Input: part model. Units: mm. Frame: model coordinates. A direction names the side the tool comes from. Coordinates: 2 decimals unless noted, no trailing zeros. Write each loop counter-clockwise with the first axis right and the second up, starting at its lowest first coordinate (ties: lowest second). Pieces come first, ordered by that corner, then holes. Notation, with made-up numbers: (40.25, 19) -> (96.25, 19) arc R14 ccw to (96.25, 38) -> close; hole circle Ø2 at (-15.5, 50). An arc over 180 degrees is marked (long way). One line per question, with ' | ' between items. Start each with the question number.
```python
from build123d import *


with BuildPart() as f1:
    # F0 (on Front) → F1 (revolve)
    with BuildSketch(Plane.XZ):
        with BuildLine():
            Line((0, 1), (0, 0))
            Line((0, 0), (6, 0))
            ThreePointArc((6, 0), (7.5, 2.5), (6, 5))
            ThreePointArc((6, 5), (4.5, 7.5), (6, 10))
            Line((6, 10), (6, 12))
            Line((6, 12), (2.75, 12))
            Line((2.75, 12), (2.75, 1))
            Line((2.75, 1), (0, 1))
        make_face()
    revolve(axis=Axis((0, 0, 0.5), (0, 0, -1)))


solid = f1.part
```
1) Ray query, line 1 (X direction, y = 2, z = 2); line 2 (X direction, y = 0, z = 9.25); line 3 (Y direction, x = 0, z = 7.5). Return the intervals inside material, ascending.
2) Access query for faces 4 (the face through (0, 0, 1)), 5 (the face through (3, 1, 12)). Directions: +Z, -Z, +X, -X, +Y, -Y. A direction counts if a zero-diameter tool reaches every point of the face in a straight line with its end or side. Return the directions, or none.
3) Section B-B, the plane z = 4.5. Return loops of the section in (x, y), then the cut area to 3 significant figures.
4) Section A-A, the plane z = 2.5. Return loops of the section in (x, y).
5) First-contact query: P1, Ø6, axis at x = 1, y = -0.5, coming from the +Z side; P2, Ø6, axis at y = 2.5, z = 5.5, coming from the +X side; P3, Ø3, axis at x = -3, z = 10.5, coming from the -Y side. Flat tips, straight axial feed; report the tip coordinate or a pass-through.
6) Pull-direction query (X, two-part tool) for faces 1 (the face through (0, 0, 0)), 2 (the face through (-6, 0, 11)), 3 (the face through (-0.596, 2.685, 6.423)); classes: released by +X, released by -X, zero draft, split by the parting line, or undercut.
Answer block:
1) line 1: x = -7.18 to -1.89, 1.89 to 7.18 | line 2: x = -5.11 to -2.75, 2.75 to 5.11 | line 3: y = -4.5 to -2.75, 2.75 to 4.5
2) face 4: +Z | face 5: +Z, +X, -X, +Y, -Y
3) outline: circle Ø13.35 at (0, 0); hole circle Ø5.5 at (0, 0) | area: 116 mm2
4) outline: circle Ø15 at (0, 0); hole circle Ø5.5 at (0, 0)
5) P1: stops at z = 12 | P2: stops at x = 7.41 | P3: stops at y = -5.81
6) face 1: zero draft | face 2: split by the parting line | face 3: undercut
